Model file for the job. Use its own axes, mm. A direction names the side the tool comes from. Coordinates: 2 decimals unless noted, no trailing zeros. Loops run counter-clockwise (first coordinate to the right, second up) from the corner with the lowest first, then second, coordinate; pieces in that order, holes last.
from build123d import *

# Parameters (mm, degrees)
BOSS_EXTRUDE1_DEPTH = 120
BOSS_EXTRUDE2_DEPTH = 98
BOSS_EXTRUDE3_DEPTH = 10
BOSS_EXTRUDE4_DEPTH = 10
FILLET5_R           = 2
FILLET6_R           = 2
SKETCH2_R           = 2.5
CUT_EXTRUDE1_DEPTH  = 100


with BuildPart() as part:
    # Sketch1 → Boss-Extrude1 (new body)
    with BuildSketch(Plane.XY):
        with BuildLine():
            Line((-24.852244642, 0), (-32.852244642, 0))
            Line((-32.852244642, 0), (-40.852244642, 0))
            ThreePointArc((-40.852244642, 0), (-32.852244642, -8), (-24.852244642, 0))
        make_face()
        with BuildLine():
            Line((-40.852244642, 0), (-32.852244642, 0))
            Line((-32.852244642, 0), (-24.852244642, 0))
            ThreePointArc((-24.852244642, 0), (-32.852244642, 8), (-40.852244642, 0))
        make_face()
    extrude(amount=BOSS_EXTRUDE1_DEPTH)

    # Sketch1_3 → Boss-Extrude2 (add)
    with BuildSketch(Plane.XY):
        with BuildLine():
            ThreePointArc((-24.852244642, 0), (-32.852244642, -8), (-40.852244642, 0))
            Line((-40.852244642, 0), (-43.852244642, 0))
            ThreePointArc((-43.852244642, 0), (-32.852244642, -11), (-21.852244642, 0))
            Line((-21.852244642, 0), (-24.852244642, 0))
        make_face()
        with BuildLine():
            Line((-43.852244642, 0), (-40.852244642, 0))
            ThreePointArc((-40.852244642, 0), (-32.852244642, 8), (-24.852244642, 0))
            Line((-24.852244642, 0), (-21.852244642, 0))
            ThreePointArc((-21.852244642, 0), (-32.852244642, 11), (-43.852244642, 0))
        make_face()
    extrude(amount=BOSS_EXTRUDE2_DEPTH)

    # Sketch1_4 → Boss-Extrude3 (add)
    with BuildSketch(Plane.XY):
        with BuildLine():
            Line((-47.852244642, 0), (-43.852244642, 0))
            ThreePointArc((-43.852244642, 0), (-32.852244642, 11), (-21.852244642, 0))
            Line((-21.852244642, 0), (-17.852244642, 0))
            Line((-17.852244642, 0), (-17.852244642, 9.949874371))
            ThreePointArc((-17.852244642, 9.949874371), (-32.852244642, 18), (-47.852244642, 9.949874371))
            Line((-47.852244642, 9.949874371), (-47.852244642, 0))
        make_face()
        with BuildLine():
            ThreePointArc((-21.852244642, 0), (-32.852244642, -11), (-43.852244642, 0))
            Line((-43.852244642, 0), (-47.852244642, 0))
            Line((-47.852244642, 0), (-47.852244642, -9.949874371))
            ThreePointArc((-47.852244642, -9.949874371), (-32.852244642, -18), (-17.852244642, -9.949874371))
            Line((-17.852244642, -9.949874371), (-17.852244642, 0))
            Line((-17.852244642, 0), (-21.852244642, 0))
        make_face()
    extrude(amount=BOSS_EXTRUDE3_DEPTH)

    # Sketch1_6 → Boss-Extrude4 (add)
    with BuildSketch(Plane.XY):
        with BuildLine():
            Line((-47.852244642, 11.66190379), (-47.852244642, 9.949874371))
            ThreePointArc((-47.852244642, 9.949874371), (-32.852244642, 18), (-17.852244642, 9.949874371))
            Line((-17.852244642, 9.949874371), (-17.852244642, 11.66190379))
            ThreePointArc((-17.852244642, 11.66190379), (-32.852244642, 19), (-47.852244642, 11.66190379))
        make_face()
        with BuildLine():
            ThreePointArc((-17.852244642, -9.949874371), (-32.852244642, -18), (-47.852244642, -9.949874371))
            Line((-47.852244642, -9.949874371), (-47.852244642, -11.66190379))
            ThreePointArc((-47.852244642, -11.66190379), (-32.852244642, -19), (-17.852244642, -11.66190379))
            Line((-17.852244642, -11.66190379), (-17.852244642, -9.949874371))
        make_face()
    extrude(amount=BOSS_EXTRUDE4_DEPTH)

    # Fillet5
    fillet5_edges = [part.edges().sort_by_distance(p)[0] for p in [
        (-17.852244642, 0, 0),
        (-47.852244642, 0, 0),
        (-32.852244642, 19, 0),
        (-32.852244642, -19, 0),
    ]]
    fillet(fillet5_edges, radius=FILLET5_R)

    # Fillet6
    fillet6_edges = [part.edges().sort_by_distance(p)[0] for p in [
        (-40.852244642, 0, 120),
    ]]
    fillet(fillet6_edges, radius=FILLET6_R)

    # Sketch2 → Cut-Extrude1 (cut)
    with BuildSketch(Plane(origin=(0, 11, 0), x_dir=(1, 0, 0), z_dir=(0, 1, 0))):
        with Locations((-32.852244642, -30)):
            Circle(SKETCH2_R)
    extrude(amount=-CUT_EXTRUDE1_DEPTH, mode=Mode.SUBTRACT)


solid = part.part
Q1. Drill centre lines: line 1 (Z direction, x = -21, y = 2.5); line 2 (X direction, y = 0.5, z = 38); line 3 (X direction, y = -2, z = 30). Where is each one in solid material? Low to high.
Answers:
line 1: z = 0 to 10
line 2: x = -43.84 to -21.86
line 3: x = -43.67 to -35.35, -30.35 to -22.04
Q2. Slice it at B-B (z = 103). List the corners of the cut face in (x, y), and give its area (3 significant figures).
Answers:
outline: circle Ø16 at (-32.85, 0)
area: 201 mm2
Q3. Mould opens along Z. For faces 1 (the cylindrical face through (-18.454, -0.163, 0.57)), 2 (the flat face through (-40, 9, 10)), 3 (the cylindrical face through (-35.35, 0.15, 29.89)) say: +Z half, -Z half, draft (parallel to the pull), parting line (faces both ways), or undercut.
Answers:
face 1: -Z half
face 2: +Z half
face 3: undercut
Q4. Which spindle directions (+Z, -Z, +X, -X, +Y, -Y) get a long thin tool onto all of the face, cutting with end or side? Do faces 4 (the cylindrical face through (-22.36, 3.3, 53.38)), 5 (the cylindrical face through (-33, -19, 6)). Say none if no direction does.
Answers:
face 4: +Z
face 5: +Z, -Z, -Y
Q5. Slice it at A-A (y = 0). List the corners of the cut face in (x, z).
Answers:
outline: (-47.85, 2) arc R2 ccw to (-45.85, 0) - (-19.85, 0) arc R2 ccw to (-17.85, 2) - (-17.85, 10) - (-21.85, 10) - (-21.85, 98) - (-24.85, 98) - (-24.85, 118) arc R2 ccw to (-26.85, 120) - (-38.85, 120) arc R2 ccw to (-40.85, 118) - (-40.85, 98) - (-43.85, 98) - (-43.85, 10) - (-47.85, 10) - close; hole circle Ø5 at (-32.85, 30)
Q6. Slice it at C-C (z = 30). List the corners of the cut face in (x, y).
Answers:
outline: (-35.35, -10.71) - (-35.35, 10.71) arc R11 ccw to start; (-30.35, -10.71) arc R11 ccw to (-30.35, 10.71) - close
Q7. Flat gauge pins, fed straight in: P1, Ø2, axis at y = 7, z = 15.5, coming from the -X side; P2, Ø2, axis at x = -22.5, z = 73, coming from the +Y side; P3, Ø5, axis at x = -26.5, z = 80, coming from the +Y side; P4, Ø3, axis at x = -32.85, z = 30, coming from the -Y side. Where does each tip first touch, or does it go through?
Answers:
P1: stops at x = -42.07
P2: stops at y = 5.79
P3: stops at y = 10.3
P4: passes through
